Print and shaded views of the part. All mm, measured from the part's lowest x, y and z. A direction names the side the tool comes from. Give positions to 0.01 mm unless a question says otherwise; leave off trailing zeros. Loops run counter-clockwise (first coordinate to the right, second up) from the corner with the lowest first, then second, coordinate; pieces in that order, holes last. Notation, with made-up numbers: M -6.5,66.5 L 26.5,66.5 A29 cw 26.5,86.5 Z; hole C 47,-33 d1. An arc over 180 degrees is marked long. Answer in a Markdown table with one row per item.
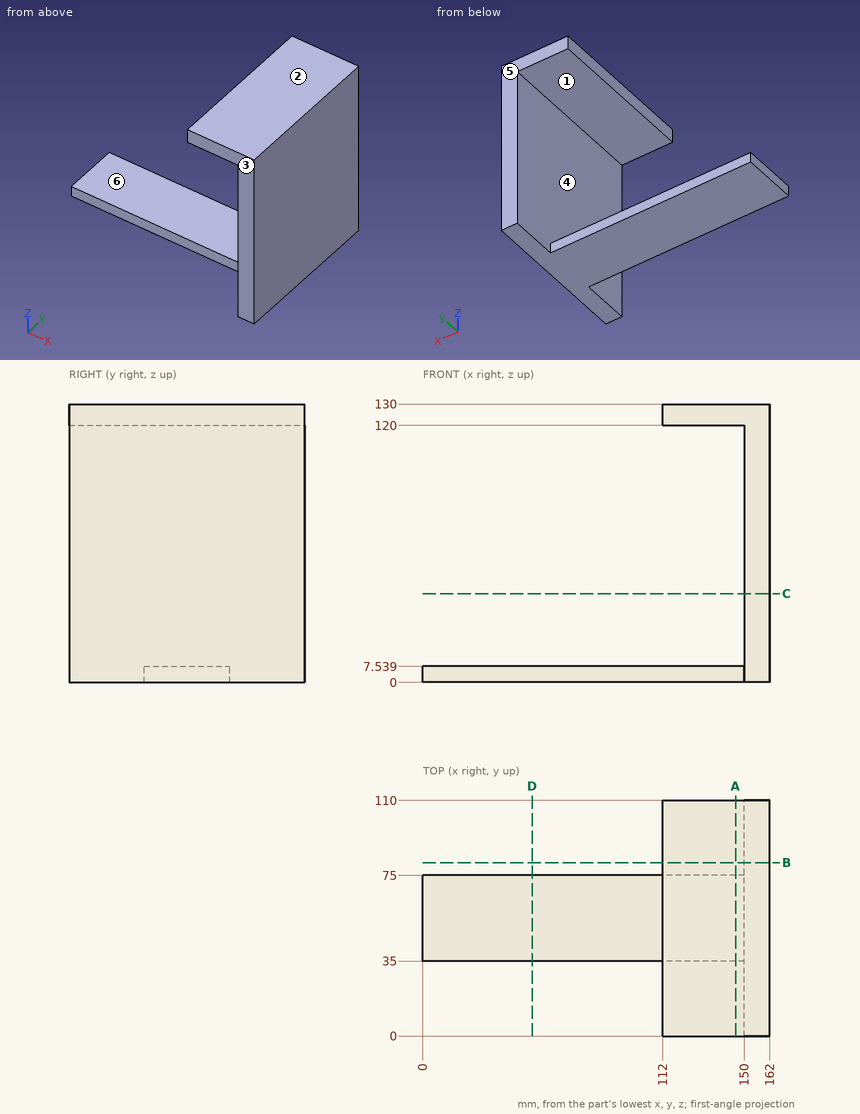
(1) Which spindle directions (+Z, -Z, +X, -X, +Y, -Y) get a long thin tool onto all of the face, cutting with end or side? Do the marked faces 5 and 6. Say none if no direction does.
Established:
| item | result |
|---|---|
| face 5 | +Z, -Z, +X, -X, +Y |
| face 6 | -X, +Y, -Y |
(2) Flat gauge pins, fed straight in: P1, Ø1, axis at y = 92, z = 22.5, coming from the -X side; P2, Ø11, axis at y = 72.5, z = 122.5, coming from the -X side; P3, Ø5, axis at x = 111.5, y = 93, coming from the -Z side. Where does each tip first touch, or does it go through?
Established:
| item | result |
|---|---|
| P1 | stops at x = 150 |
| P2 | stops at x = 112 |
| P3 | stops at z = 120 |
(3) Saw through at B-B, the plane y = 81. Give the cut face in (x, z), and give its area (3 significant figures).
Established:
| item | result |
|---|---|
| outline | M 112,120 L 150,120 L 150,0 L 162,0 L 162,130 L 112,130 Z |
| area | 1,940 mm2 |
(4) Mould opens along Z. For the marked faces 1, 2, 3 and 4 say: pulls with the +Z half, pulls with the -Z half, needs draft (parallel to the pull), parting line crosses it, or undercut.
Established:
| item | result |
|---|---|
| face 1 | undercut |
| face 2 | pulls with the +Z half |
| face 3 | needs draft |
| face 4 | undercut |
(5) Wall check: L1, parallel to X at y = 42, z = 15; L2, parallel to Z at x = 126.5, y = 17; L3, parallel to Z at x = 105.5, y = 69.5. Give the ranges that are in metal, low to high.
Established:
| item | result |
|---|---|
| L1 | x = 150 to 162 |
| L2 | z = 120 to 130 |
| L3 | z = 0 to 7.54 |
(6) Saw through at C-C, the plane z = 41.5. Give the cut face in (x, y).
Established:
| item | result |
|---|---|
| outline | M 150,0 L 162,0 L 162,110 L 150,110 Z |
(7) Saw through at D-D, the plane x = 51. Give the cut face in (y, z).
Established:
| item | result |
|---|---|
| outline | M 35,0 L 75,0 L 75,7.54 L 35,7.54 Z |
(8) Saw through at A-A, the plane x = 146. Give the cut face in (y, z).
Established:
| item | result |
|---|---|
| outline | M 0,120 L 110,120 L 110,130 L 0,130 Z; M 35,0 L 75,0 L 75,7.54 L 35,7.54 Z |
